```python
from build123d import *

# Parameters (mm, degrees)
F1_DEPTH = 25.4
F2_R     = 139.7
F3_DEPTH = 25.4
F4_R     = 3.175
F5_DEPTH = 25.401


with BuildPart() as f1:
    # F0 (on Top) → F1 (new body)
    with BuildSketch(Plane.XY):
        with BuildLine():
            Line((-152.4, -177.8), (152.4, -177.8))
            ThreePointArc((152.4, -177.8), (170.360512, -170.360512), (177.8, -152.4))
            Line((177.8, -152.4), (177.8, 152.4))
            ThreePointArc((177.8, 152.4), (170.360512, 170.360512), (152.4, 177.8))
            Line((152.4, 177.8), (-152.4, 177.8))
            ThreePointArc((-152.4, 177.8), (-170.360512, 170.360512), (-177.8, 152.4))
            Line((-177.8, 152.4), (-177.8, -152.4))
            ThreePointArc((-177.8, -152.4), (-170.360512, -170.360512), (-152.4, -177.8))
        make_face()
    extrude(amount=F1_DEPTH)

    # F2 (on face) → F3 (cut)
    with BuildSketch(Plane.XY.offset(25.4)):
        Circle(F2_R)
    extrude(amount=-F3_DEPTH, mode=Mode.SUBTRACT)

    # F4 (on face) → F5 (cut, through all)
    with BuildSketch(Plane.XY.offset(25.4)):
        with Locations((-148.683629, 12.699569)):
            Circle(F4_R)
        with Locations((-148.839737, -10.716028)):
            Circle(F4_R)
        with Locations((-145.330917, -33.867761)):
            Circle(F4_R)
        with Locations((-138.243567, -56.185557)):
            Circle(F4_R)
        with Locations((-127.752202, -77.119878)):
            Circle(F4_R)
        with Locations((-114.115153, -96.155251)):
            Circle(F4_R)
        with Locations((-97.668211, -112.822964)):
            Circle(F4_R)
        with Locations((-78.816354, -126.7126)):
            Circle(F4_R)
        with Locations((-58.023776, -137.482152)):
            Circle(F4_R)
        with Locations((-35.80246, -144.866437)):
            Circle(F4_R)
        with Locations((-12.699569, -148.683629)):
            Circle(F4_R)
        with Locations((10.716028, -148.839737)):
            Circle(F4_R)
        with Locations((33.867761, -145.330917)):
            Circle(F4_R)
        with Locations((56.185557, -138.243567)):
            Circle(F4_R)
        with Locations((77.119878, -127.752202)):
            Circle(F4_R)
        with Locations((96.155251, -114.115153)):
            Circle(F4_R)
        with Locations((112.822964, -97.668211)):
            Circle(F4_R)
        with Locations((126.7126, -78.816354)):
            Circle(F4_R)
        with Locations((137.482152, -58.023776)):
            Circle(F4_R)
        with Locations((144.866437, -35.80246)):
            Circle(F4_R)
        with Locations((148.683629, -12.699569)):
            Circle(F4_R)
        with Locations((148.839737, 10.716028)):
            Circle(F4_R)
        with Locations((145.330917, 33.867761)):
            Circle(F4_R)
        with Locations((138.243567, 56.185557)):
            Circle(F4_R)
        with Locations((127.752202, 77.119878)):
            Circle(F4_R)
        with Locations((114.115153, 96.155251)):
            Circle(F4_R)
        with Locations((97.668211, 112.822964)):
            Circle(F4_R)
        with Locations((78.816354, 126.7126)):
            Circle(F4_R)
        with Locations((58.023776, 137.482152)):
            Circle(F4_R)
        with Locations((35.80246, 144.866437)):
            Circle(F4_R)
        with Locations((12.699569, 148.683629)):
            Circle(F4_R)
        with Locations((-10.716028, 148.839737)):
            Circle(F4_R)
        with Locations((-33.867761, 145.330917)):
            Circle(F4_R)
        with Locations((-56.185557, 138.243567)):
            Circle(F4_R)
        with Locations((-77.119878, 127.752202)):
            Circle(F4_R)
        with Locations((-96.155251, 114.115153)):
            Circle(F4_R)
        with Locations((-112.822964, 97.668211)):
            Circle(F4_R)
        with Locations((-126.7126, 78.816354)):
            Circle(F4_R)
        with Locations((-137.482152, 58.023776)):
            Circle(F4_R)
        with Locations((-144.866437, 35.80246)):
            Circle(F4_R)
    extrude(amount=-F5_DEPTH, mode=Mode.SUBTRACT)


solid = f1.part
```
Read the model definition and answer for the solid it produces. Units are mm, in the model's axes. Give positions to 0.01 mm unless a question says otherwise; leave off trailing zeros. Write each loop counter-clockwise with the first axis right and the second up, starting at its lowest first coordinate (ties: lowest second). Pieces come first, ordered by that corner, then holes. Notation, with made-up numbers: M 25,-39 L 48,-39 A13 ccw 48,-18 Z; hole C 6.5,48 d5. An arc over 180 degrees is marked long. Put each result on its own line as item: value. Start each with the question number.
1. Consider line 1 along X through (y, z) = (80, 13); line 2 along Y through (x, z) = (114.5, 16); line 3 along Y through (x, z) = (35, 4.5). Determine where each line is inside the solid, lowest interval first.
2. Each of these flat-tipped pins is pushed along its axis until it touches: pin 1 Ø7.5 at (x, y) = (10.72, -148.84) entering from +Z; pin 2 Ø5 at (x, y) = (148.68, -12.7) entering from +Z. Where does it stop, or does it pass through?
3. For a pull along Y with two mould halves and no side action, classify faces 1 (the cylindrical face through (-170.56, -170.16, 12.52)), 2 (the cylindrical face through (-110.86, -85.01, 12.88)), 3 (the cylindrical face through (-170.16, 170.56, 12.52)), 4 (the flat face through (-177.8, 2, 13)) as released by +Y, released by -Y, zero draft, split by the parting line, or undercut.
4. The part is cut by section A-A, the plane x = 0. Give the vertices of the cut face in (y, z).
5. The part is cut by section C-C, the plane z = 15.5. Give the number of separate pieces and of enclosed holes in the cut face, and give its area (3 significant figures).
Final values:
1. line 1: x = -177.8 to -129.66, -123.77 to -114.53, 114.53 to 126.42, 129.09 to 177.8
1. line 2: y = -177.8 to -100.36, -94.97 to -80.04, 80.04 to 93, 99.31 to 177.8
1. line 3: y = -177.8 to -148.3, -142.36 to -135.24, 135.24 to 141.79, 147.94 to 177.8
2. pin 1: stops at z = 25.4
2. pin 2: passes through
3. face 1: released by -Y
3. face 2: undercut
3. face 3: released by +Y
3. face 4: zero draft
4. outline: M -177.8,0 L -139.7,0 L -139.7,25.4 L -177.8,25.4 Z; M 139.7,0 L 177.8,0 L 177.8,25.4 L 139.7,25.4 Z
5. separate pieces: 1
5. enclosed holes: 41
5. area: 63,300 mm²
